Here's how the part is built. I have some questions about the finished solid (model axes, mm). A direction names the side the tool comes from. Give positions to 0.01 mm unless a question says otherwise; leave off trailing zeros. Loops run counter-clockwise (first coordinate to the right, second up) from the corner with the lowest first, then second, coordinate; pieces in that order, holes last. Notation, with made-up numbers: (-2, -34) -> (40, -34) arc R30 cw to (40, 2) -> close; hole circle Ø10 at (-28, 35). An arc over 180 degrees is marked (long way). Answer in a Markdown table with one row per item. Add a question column.
Item 1: If we section it at A-A (x = -35): Write out the boundary of the cut face in (y, z).
Item 2: If I drill on line 1 (Y direction, x = -35, z = 23); line 2 (Z direction, x = -73.5, y = -9); line 3 (Z direction, x = -100, y = -35), over which ranges is the centre line in solid material (lowest first)?
Item 3: We'd pull the mould along X, two halves only. Please class faces 1 (the face through (-16.954, 10.84, 12.362)), 2 (the face through (-114.456, 10.84, 10.14)), 3 (the face through (-43, 0, 17)): released by +X, released by -X, zero draft, split by the parting line, or undercut.
Item 4: Which directions (+Z, -Z, +X, -X, +Y, -Y) give clear straight access to the entire face, cutting with the end or side of a thin tool? Please do faces 4 (the face through (-99, -29.416, 37)), 5 (the face through (-83.295, -23, 37)), 6 (the face through (-99, -16.273, 37)), 7 (the face through (-115.201, -23, 37)).
Item 5: For P1, Ø8, axis at x = -34.5, y = 20, coming from the -Z side; P2, Ø7.5, axis at x = -91.5, z = 39, coming from the -Y side; P3, Ø1.5, axis at x = -74.5, z = 15, coming from the -Y side; P4, Ø20, axis at x = -97, z = 34, coming from the +Y side, each with a flat end and sliding along its axis, tell me the tip position at first contact or that it passes through.
Item 6: If we section it at D-D (z = 18.5): Write out the boundary of the cut face in (x, y).
Item 7: If we section it at B-B (y = 0): Write out the boundary of the cut face in (x, z).
Item 8: If we section it at C-C (x = -86.5): Write out the boundary of the cut face in (y, z).
```python
from build123d import *

# Parameters (mm, degrees)
F0_W        = 115
F0_H        = 120
F0_R        = 5
F1_DEPTH    = 25
F2_W        = 31.9062322378
F2_H        = 13.1420847028
F3_DEPTH    = 25
F4_T1_DEPTH = 217.8673195186
F4_T3_DEPTH = 222.8673195186


# Not quite as in the source:
# - a fillet or chamfer that OpenCascade refuses, or shapes differently, is made with other operations: its cross-section is extruded or revolved along the edge and cut away or added


with BuildPart() as f1:
    # F0 (on Top) → F1 (new body)
    with BuildSketch(Plane.XY):
        with Locations((-66.8158578873, 10)):
            Rectangle(F0_W, F0_H)
        with Locations((-35, 0)):
            Circle(F0_R, mode=Mode.SUBTRACT)
    extrude(amount=F1_DEPTH)

    # F2 (on face) → F3 (join)
    with BuildSketch(Plane.XY.offset(25)):
        with Locations((-99.2479249835, -22.8444887325)):
            Rectangle(F2_W, F2_H)
    extrude(amount=F3_DEPTH)

    # F4: chamfer of 20 on 5 edges, made by hand

    # F4_s2 → F4_t1 (cut)
    with BuildSketch(Plane.YZ.offset(-175.7495176466)):
        Polygon((-50, 20), (-30, 0), (-50, 0), align=None)
        Polygon((50, 0), (70, 20), (70, 0), align=None)
    extrude(amount=F4_T1_DEPTH, mode=Mode.SUBTRACT)

    # F4_s4 → F4_t3 (cut)
    with BuildSketch(Plane.XZ.offset(-121.4336597593)):
        Polygon((-9.3158578873, 20), (-29.3158578873, 0), (-9.3158578873, 0), align=None)
        Polygon((-124.3158578873, 20), (-104.3158578873, 0), (-124.3158578873, 0), align=None)
    extrude(amount=F4_T3_DEPTH, mode=Mode.SUBTRACT)

    # F4_s5 → F4_t6 (revolve, cut)
    with BuildSketch(Plane.XZ):
        Polygon((-10, 0), (-30, 20), (-30, 0), align=None)
    revolve(axis=Axis((-35, 0, 0), (0, 0, 1)), mode=Mode.SUBTRACT)


solid = f1.part
```
Recorded:
| question | item | result |
|---|---|---|
| 1 | outline | (-50, 20) -> (-30, 0) -> (-25, 0) -> (-5, 20) -> (-5, 25) -> (-50, 25) -> close; (5, 20) -> (25, 0) -> (50, 0) -> (70, 20) -> (70, 25) -> (5, 25) -> close |
| 2 | line 1 | y = -50 to -5, 5 to 70 |
| 2 | line 2 | z = 0 to 25 |
| 2 | line 3 | z = 5 to 25 |
| 3 | face 1 | released by +X |
| 3 | face 2 | released by -X |
| 3 | face 3 | undercut |
| 4 | face 4 | +Z, +X, -X, -Y |
| 4 | face 5 | +Z, +X, +Y, -Y |
| 4 | face 6 | +Z, +X, -X, +Y |
| 4 | face 7 | +Z, -X, +Y, -Y |
| 5 | P1 | stops at z = 0.99 |
| 5 | P2 | stops at y = -29.42 |
| 5 | P3 | stops at y = -45.75 |
| 5 | P4 | stops at y = 70 |
| 6 | outline | (-122.82, -48.5) -> (-10.82, -48.5) -> (-10.82, 68.5) -> (-122.82, 68.5) -> close; hole circle Ø13 at (-35, 0) |
| 7 | outline | (-124.32, 20) -> (-104.32, 0) -> (-60, 0) -> (-40, 20) -> (-40, 25) -> (-124.32, 25) -> close; (-30, 20) -> (-19.66, 9.66) -> (-9.32, 20) -> (-9.32, 25) -> (-30, 25) -> close |
| 8 | outline | (-50, 20) -> (-30, 0) -> (50, 0) -> (70, 20) -> (70, 25) -> (-16.27, 25) -> (-16.27, 50) -> (-29.42, 50) -> (-29.42, 25) -> (-50, 25) -> close |
